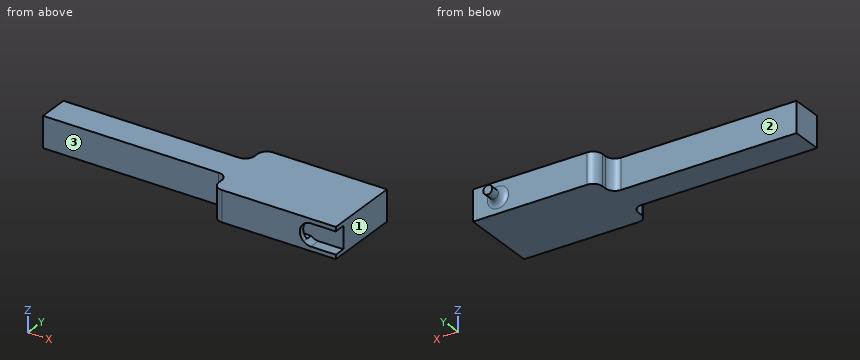
```python
from build123d import *

# Parameters (mm, degrees)
SKETCH2_W               = 100
SKETCH2_H               = 10
BOSS_EXTRUDE2_DEPTH     = 12.5
CAVITY1_START           = -10.85
CAVITY1_OUTLINE_R       = 1.325
CAVITY1_DEPTH           = 2
CAVITY1_START_2         = -12.5
CAVITY1_2_OUTLINE_R     = 2.1
CAVITY1_2_DEPTH         = 1.65
CUT_EXTRUDE1_START      = -3.65
SKETCH3_R               = 2.1
CUT_EXTRUDE1_DEPTH      = 3.65
SKETCH4_W               = 8.1
SKETCH4_H               = 7.2
CUT_EXTRUDE2_DEPTH      = 3.65
SKETCH5_R               = 1.45
BOSS_EXTRUDE3_DEPTH     = 5
FILLET1_R               = 2
CUT_EXTRUDE3_DEPTH      = 54.909646632
CUT_EXTRUDE3_DEPTH_BACK = 54.909646632
SKETCH6_W               = 60
SKETCH6_H               = 7.5
FILLET2_R               = 3


# Read off the part's stored shape, not the designer's step: Cavity1
with BuildPart() as part:
    # Sketch2 → Boss-Extrude2 (new, symmetric)
    with BuildSketch(Plane(origin=(0, 0, 0), x_dir=(1, 0, 0), z_dir=(0, 1, 0))):
        Rectangle(SKETCH2_W, SKETCH2_H)
    extrude(amount=BOSS_EXTRUDE2_DEPTH, both=True)

    # Cavity1 outline → Cavity1 (cut)
    with BuildSketch(Plane(origin=(0, 0, 0), x_dir=(1, 0, 0), z_dir=(0, 1, 0)).offset(CAVITY1_START)):
        with BuildLine():
            Line((26.51882382, -2.1), (39.51882382, -2.7))
            ThreePointArc((39.51882382, -2.7), (45.5, 0), (39.51882382, 2.7))
            Line((39.51882382, 2.7), (26.51882382, 2.1))
            ThreePointArc((26.51882382, 2.1), (24.41882382, 0), (26.51882382, -2.1))
        make_face()
        with Locations((41.9, 0)):
            Circle(CAVITY1_OUTLINE_R, mode=Mode.SUBTRACT)
    extrude(amount=CAVITY1_DEPTH, mode=Mode.SUBTRACT)

    # Cavity1 2 outline → Cavity1 2 (cut)
    with BuildSketch(Plane(origin=(0, 0, 0), x_dir=(1, 0, 0), z_dir=(0, 1, 0)).offset(CAVITY1_START_2)):
        with BuildLine():
            ThreePointArc((39.51882382, -2.7), (45.5, 0), (39.51882382, 2.7))
            ThreePointArc((39.51882382, 2.7), (38.320838024, 0), (39.51882382, -2.7))
        make_face()
        with Locations((41.9, 0)):
            Circle(CAVITY1_2_OUTLINE_R, mode=Mode.SUBTRACT)
    extrude(amount=CAVITY1_2_DEPTH, mode=Mode.SUBTRACT)

    # Sketch3 → Cut-Extrude1 (cut)
    with BuildSketch(Plane.XZ.offset(12.5).offset(CUT_EXTRUDE1_START)):
        with Locations((41.9, 0)):
            Circle(SKETCH3_R)
    extrude(amount=CUT_EXTRUDE1_DEPTH, mode=Mode.SUBTRACT)

    # Sketch4 → Cut-Extrude2 (cut)
    with BuildSketch(Plane.XZ.offset(8.85)):
        with Locations((45.95, 0)):
            Rectangle(SKETCH4_W, SKETCH4_H)
    extrude(amount=CUT_EXTRUDE2_DEPTH, mode=Mode.SUBTRACT)

    # Sketch5 → Boss-Extrude3 (add)
    with BuildSketch(Plane(origin=(0, 12.5, 0), x_dir=(1, 0, 0), z_dir=(0, 1, 0))):
        with Locations(Location((41.9, 0, 0), (0, 0, 90))):
            Circle(SKETCH5_R)
    extrude(amount=BOSS_EXTRUDE3_DEPTH)

    # Fillet1
    fillet1_edges = [part.edges().sort_by_distance(p)[0] for p in [
        (41.9, 12.5, 1.45),
    ]]
    fillet(fillet1_edges, radius=FILLET1_R)

    # Sketch6 → Cut-Extrude3 (cut, two sides: drawn at the far end of the back side and taken through both)
    with BuildSketch(Plane.XY.offset(5).offset(-CUT_EXTRUDE3_DEPTH_BACK)):
        with Locations((-20, 8.75)):
            Rectangle(SKETCH6_W, SKETCH6_H)
        with Locations((-20, -8.75)):
            Rectangle(SKETCH6_W, SKETCH6_H)
    extrude(amount=CUT_EXTRUDE3_DEPTH + CUT_EXTRUDE3_DEPTH_BACK, mode=Mode.SUBTRACT)

    # Fillet2
    fillet2_edges = [part.edges().sort_by_distance(p)[0] for p in [
        (10, 5, 0),
        (10, 12.5, 0),
        (10, -12.5, 0),
        (10, -5, 0),
    ]]
    fillet(fillet2_edges, radius=FILLET2_R)


solid = part.part
```
For this review, take the finished solid that the model builds, in its own axes (mm). Face numbers are marked on the shaded views. A direction names the side the tool comes from. Coordinates: 2 decimals unless noted, no trailing zeros. Loops run counter-clockwise (first coordinate to the right, second up) from the corner with the lowest first, then second, coordinate; pieces in that order, holes last.
1. Add section C-C, the plane x = 21.5. Give the boundary of the cut face in (y, z).
2. Add section A-A, the plane z = 0. Give the boundary of the cut face in (x, y).
3. For the marked faces 1, 2 and 3, list the 3-axis set-ups (+Z, -Z, +X, -X, +Y, -Y) from which the entire face can be reached by the end or side of a thin tool; tool diameter is ignored.
4. For line 1 (Y direction, x = 35, z = 3.75); line 2 (Y direction, x = -10.5, z = -1); line 3 (X direction, y = 7.75, z = 0.75), list the stretches that pass through material, from the lowest coordinate up.
5. Add section B-B, the plane x = -42. Give the boundary of the cut face in (y, z).
6. Insertion check: P1, Ø1.2, axis at y = -9, z = -0.5, coming from the -X side; P2, Ø4, axis at x = 7.5, z = 4, coming from the -Y side; P3, Ø4.5, axis at x = 34, z = 0.5, coming from the +Y side. Each pin has a flat end and moves straight along its axis. Give the tip position at first contact, or say it passes through.
Result:
1. outline: (-12.5, -5) - (12.5, -5) - (12.5, 5) - (-12.5, 5) - close
2. outline: (-50, -5) - (7, -5) arc R3 cw to (10, -8) - (10, -9.5) arc R3 ccw to (13, -12.5) - (38.32, -12.5) - (38.32, -10.85) - (24.42, -10.85) - (24.42, -8.85) - (50, -8.85) - (50, 12.5) - (45.35, 12.5) arc R2 cw to (43.35, 14.5) - (43.35, 17.5) - (40.45, 17.5) - (40.45, 14.5) arc R2 cw to (38.45, 12.5) - (13, 12.5) arc R3 ccw to (10, 9.5) - (10, 8) arc R3 cw to (7, 5) - (-50, 5) - close
3. face 1: +Z, -Z, +X, +Y, -Y
3. face 2: +Z, -Z, -X, +Y
3. face 3: +Z, -Z, -X, -Y
4. line 1: y = -12.5 to 12.5
4. line 2: y = -5 to 5
4. line 3: x = 9.99 to 50
5. outline: (-5, -5) - (5, -5) - (5, 5) - (-5, 5) - close
6. P1: stops at x = 10
6. P2: stops at y = -6.34
6. P3: stops at y = 12.5
